from build123d import *

# Parameters (mm, degrees)
F0_W     = 50
F0_H     = 50
F1_DEPTH = 400
F2_START = 400
F0_H_2   = 400
F0_W_2   = 400
F2_DEPTH = 50
F3_START = 450
F3_DEPTH = 100
F4_START = 550
F4_DEPTH = 350


with BuildPart() as f1:
    # F0 (on Top) → F1 (new body)
    with BuildSketch(Plane.XY):
        with Locations((225, 225)):
            Rectangle(F0_W, F0_H)
    extrude(amount=F1_DEPTH)



with BuildPart() as f1b:
    # F0 (on Top) → F1, piece 2 (new body)
    with BuildSketch(Plane.XY):
        with Locations((-225, 225)):
            Rectangle(F0_W, F0_H)
    extrude(amount=F1_DEPTH)


with BuildPart() as f1c:
    # F0 (on Top) → F1, piece 3 (new body)
    with BuildSketch(Plane.XY):
        with Locations((-225, -225)):
            Rectangle(F0_W, F0_H)
    extrude(amount=F1_DEPTH)


with BuildPart() as f1d:
    # F0 (on Top) → F1, piece 4 (new body)
    with BuildSketch(Plane.XY):
        with Locations((225, -225)):
            Rectangle(F0_W, F0_H)
    extrude(amount=F1_DEPTH)


with BuildPart() as f1_1:
    add(f1.part)

    add(f1b.part)  # F2 merges F1b

    add(f1c.part)  # F2 merges F1c

    add(f1d.part)  # F2 merges F1d
    # F0 (on Top) → F2 (join)
    with BuildSketch(Plane.XY.offset(F2_START)):
        with Locations((-225, 0)):
            Rectangle(F0_W, F0_H_2)
        Rectangle(F0_W_2, F0_H_2)
        with Locations((0, 225)):
            Rectangle(F0_W_2, F0_H)
        with Locations((225, 0)):
            Rectangle(F0_W, F0_H_2)
        with Locations((0, -225)):
            Rectangle(F0_W_2, F0_H)
        with Locations((-225, -225)):
            Rectangle(F0_W, F0_H)
        with Locations((-225, 225)):
            Rectangle(F0_W, F0_H)
        with Locations((225, 225)):
            Rectangle(F0_W, F0_H)
        with Locations((225, -225)):
            Rectangle(F0_W, F0_H)
    extrude(amount=F2_DEPTH)

    # F0 (on Top) → F3 (join)
    with BuildSketch(Plane.XY.offset(F3_START)):
        with Locations((225, 225)):
            Rectangle(F0_W, F0_H)
        with Locations((-225, 225)):
            Rectangle(F0_W, F0_H)
    extrude(amount=F3_DEPTH)

    # F0 (on Top) → F4 (join)
    with BuildSketch(Plane.XY.offset(F4_START)):
        with Locations((0, 225)):
            Rectangle(F0_W_2, F0_H)
        with Locations((225, 225)):
            Rectangle(F0_W, F0_H)
        with Locations((-225, 225)):
            Rectangle(F0_W, F0_H)
    extrude(amount=F4_DEPTH)


solid = f1_1.part
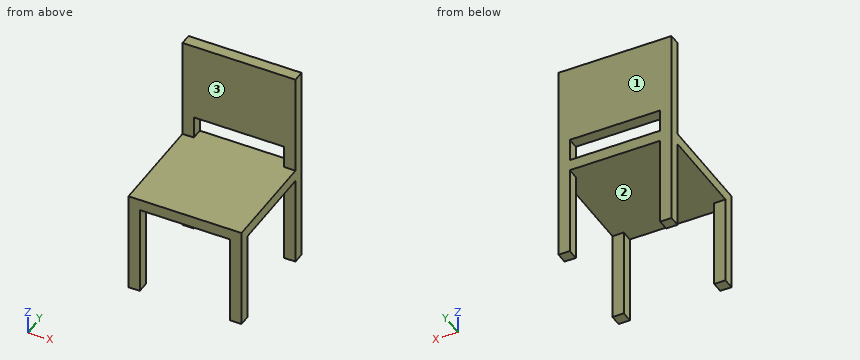
Model file for the job. Use its own axes, mm. Face numbers are marked on the shaded views. Give positions to 0.01 mm unless a question says otherwise; leave off trailing zeros. Loops run counter-clockwise (first coordinate to the right, second up) from the corner with the lowest first, then second, coordinate; pieces in that order, holes last. Notation, with made-up numbers: (38.25, -29.75) -> (97.25, -29.75) arc R9 cw to (97.25, -19.75) -> close; hole circle Ø2 at (58.5, -33). An arc over 180 degrees is marked (long way). Use a Markdown table: item, result. Add a question column.
(1) Slice it at A-A on z = 172. List the corners of the cut face in (x, y).
(2) Slice it at B-B on x = -132. List the corners of the cut face in (y, z), and give its area (3 significant figures).
(3) Mould opens along Y. For the marked faces 1, 2 and 3 say: +Y half, -Y half, draft (parallel to the pull), parting line (faces both ways), or undercut.
(4) Drop flat-ended pins along their axis: pin 1 Ø5 at (x, y) = (-164.5, -83.5) entering from -Z; pin 2 Ø10 at (x, y) = (-160, 180) entering from +Z. Give the stop position or say it passes through.
(5) Slice it at C-C on z = 780. List the corners of the cut face in (x, y), and give its area (3 significant figures).
(6) Slice it at D-D on y = -61. List the corners of the cut face in (x, z).
(7) Wall check: line 1 along Z through (x, y) = (-113, 202); line 2 along Y through (x, z) = (-224, 87.5). Give the ranges that are in metal, low to high.
Filled sheet:
| question | item | result |
|---|---|---|
| 1 | outline | (-250, -250) -> (-200, -250) -> (-200, -200) -> (-250, -200) -> close; (-250, 200) -> (-200, 200) -> (-200, 250) -> (-250, 250) -> close; (200, -250) -> (250, -250) -> (250, -200) -> (200, -200) -> close; (200, 200) -> (250, 200) -> (250, 250) -> (200, 250) -> close |
| 2 | outline | (-250, 400) -> (250, 400) -> (250, 450) -> (-250, 450) -> close; (200, 550) -> (250, 550) -> (250, 900) -> (200, 900) -> close |
| 2 | area | 42,500 mm2 |
| 3 | face 1 | +Y half |
| 3 | face 2 | undercut |
| 3 | face 3 | -Y half |
| 4 | pin 1 | z = 400 |
| 4 | pin 2 | z = 450 |
| 5 | outline | (-250, 200) -> (250, 200) -> (250, 250) -> (-250, 250) -> close |
| 5 | area | 25,000 mm2 |
| 6 | outline | (-250, 400) -> (250, 400) -> (250, 450) -> (-250, 450) -> close |
| 7 | line 1 | 400 to 450, 550 to 900 |
| 7 | line 2 | -250 to -200, 200 to 250 |
